Work out the finished part from the listing and answer in its coordinate system (mm). Face numbers are marked on the shaded views. A direction names the side the tool comes from. Give positions to 0.01 mm unless a question says otherwise; leave off trailing zeros. Order: outer loops, then holes, each group sorted by start corner. A loop starts at its lowest first (then second) coordinate and runs counter-clockwise, first axis right, second up.
```python
from build123d import *

# Parameters (mm, degrees)
CYLINDER002_R          = 2
CYLINDER002_DEPTH      = 2
CYLINDER_R             = 1.05
CYLINDER_DEPTH         = 20
CYLINDER_ROLL_ANGLE    = 90
RECTANGLE004_W         = 26
RECTANGLE004_H         = 4.8
EXTRUDE005_DEPTH       = 8
RECTANGLE002_W         = 26
RECTANGLE002_H         = 1
EXTRUDE004_DEPTH       = 20
RECTANGLE005_W         = 26
RECTANGLE005_H         = 4.8
EXTRUDE008_DEPTH       = 8
RECTANGLE001_W         = 26
RECTANGLE001_H         = 1
EXTRUDE002_DEPTH       = 20
RECTANGLE_W            = 27
RECTANGLE_H            = 15
EXTRUDE_DEPTH          = 9
FILLET_R               = 4
FILLET001_R            = 1.8
RECTANGLE008_W         = 26
RECTANGLE008_H         = 4.8
EXTRUDE011_DEPTH       = 8
RECTANGLE007_W         = 26
RECTANGLE007_H         = 1
EXTRUDE010_DEPTH       = 20
RECTANGLE009_W         = 26
RECTANGLE009_H         = 4.8
EXTRUDE012_DEPTH       = 8
RECTANGLE006_W         = 26
RECTANGLE006_H         = 1
EXTRUDE009_DEPTH       = 20
CYLINDER001_R          = 3
CYLINDER001_DEPTH      = 15
CYLINDER001_ROLL_ANGLE = 90
CUT002_ROLL_ANGLE      = 90


with BuildPart() as cylinder002:
    # Cylinder002 → Cylinder002 (new body)
    with BuildSketch(Plane(origin=(-14, -1.5, 18), x_dir=(1, 0, 0), z_dir=(0, 0, 1))):
        Circle(CYLINDER002_R)
    extrude(amount=CYLINDER002_DEPTH)


with BuildPart() as cylinder:
    # Cylinder → Cylinder (new body)
    with BuildSketch(Plane.XY):
        Circle(CYLINDER_R)
    extrude(amount=CYLINDER_DEPTH)


with BuildPart() as cylinder_1:
    # Cylinder roll: moved
    add(cylinder.part.rotate(Axis((0, 0, 0), (1, 0, 0)), CYLINDER_ROLL_ANGLE))


with BuildPart() as cylinder_2:
    # Cylinder placement: moved
    add(cylinder_1.part.moved(Location((-14, 21, 1.5))))


with BuildPart() as extrude005:
    # Rectangle004 → Extrude005 (new body)
    with BuildSketch(Plane(origin=(-23, 13.1, 0), x_dir=(1, 0, 0), z_dir=(0, 0, 1))):
        with Locations((13, 2.4)):
            Rectangle(RECTANGLE004_W, RECTANGLE004_H)
    extrude(amount=-EXTRUDE005_DEPTH)


with BuildPart() as extrude005_1:
    # Extrude005 placement: moved
    add(extrude005.part.moved(Location((0, 0, 11))))


with BuildPart() as extrude004:
    # Rectangle002 → Extrude004 (new body)
    with BuildSketch(Plane(origin=(-23, 10, 0), x_dir=(1, 0, 0), z_dir=(0, 0, 1))):
        with Locations((13, -0.5)):
            Rectangle(RECTANGLE002_W, RECTANGLE002_H)
    extrude(amount=EXTRUDE004_DEPTH)


with BuildPart() as extrude004_1:
    # Extrude004 placement: moved
    add(extrude004.part.moved(Location((0, 0, -4))))


with BuildPart() as extrude008:
    # Rectangle005 → Extrude008 (new body)
    with BuildSketch(Plane(origin=(-23, 11.9, 0), x_dir=(1, 0, 0), z_dir=(0, 0, 1))):
        with Locations((13, -2.4)):
            Rectangle(RECTANGLE005_W, RECTANGLE005_H)
    extrude(amount=EXTRUDE008_DEPTH)


with BuildPart() as extrude008_1:
    # Extrude008 placement: moved
    add(extrude008.part.moved(Location((0, 0, 3))))


with BuildPart() as fusion:
    # Rectangle001 → Extrude002 (new body)
    with BuildSketch(Plane(origin=(-23, 16, 0), x_dir=(1, 0, 0), z_dir=(0, 0, 1))):
        with Locations((13, 0.5)):
            Rectangle(RECTANGLE001_W, RECTANGLE001_H)
    extrude(amount=-EXTRUDE002_DEPTH)


with BuildPart() as fusion_1:
    # Extrude002 placement: moved
    add(fusion.part.moved(Location((0, -1, 10))))

    # Fusion: union Extrude005, Extrude004, Extrude008
    add(extrude005_1.part)
    add(extrude004_1.part)
    add(extrude008_1.part)


with BuildPart() as fillet001:
    # Rectangle → Extrude (new body)
    with BuildSketch(Plane(origin=(-20, 20, 0), x_dir=(1, 0, 0), z_dir=(0, 0, 1))):
        with Locations((13.5, -7.5)):
            Rectangle(RECTANGLE_W, RECTANGLE_H)
    extrude(amount=EXTRUDE_DEPTH)

    # Fillet
    fillet_edges = [fillet001.edges().sort_by_distance(p)[0] for p in [
        (-20, 20, 4.5),
        (7, 20, 4.5),
        (7, 5, 4.5),
        (-20, 5, 4.5),
    ]]
    fillet(fillet_edges, radius=FILLET_R)

    # Cut: cut Fusion
    add(fusion_1.part, mode=Mode.SUBTRACT)

    # Fillet001
    fillet001_edges = [fillet001.edges().sort_by_distance(p)[0] for p in [
        (-8.259972, 17.9, 3),
        (-8.259972, 7.1, 3),
        (-8.5, 11.9, 3),
        (-8.5, 13.1, 3),
    ]]
    fillet(fillet001_edges, radius=FILLET001_R)


with BuildPart() as extrude011:
    # Rectangle008 → Extrude011 (new body)
    with BuildSketch(Plane(origin=(-23, 13.1, 0), x_dir=(1, 0, 0), z_dir=(0, 0, 1))):
        with Locations((13, 2.4)):
            Rectangle(RECTANGLE008_W, RECTANGLE008_H)
    extrude(amount=-EXTRUDE011_DEPTH)


with BuildPart() as extrude011_1:
    # Extrude011 placement: moved
    add(extrude011.part.moved(Location((0, 0, 11))))


with BuildPart() as extrude010:
    # Rectangle007 → Extrude010 (new body)
    with BuildSketch(Plane(origin=(-23, 10, 0), x_dir=(1, 0, 0), z_dir=(0, 0, 1))):
        with Locations((13, -0.5)):
            Rectangle(RECTANGLE007_W, RECTANGLE007_H)
    extrude(amount=EXTRUDE010_DEPTH)


with BuildPart() as extrude010_1:
    # Extrude010 placement: moved
    add(extrude010.part.moved(Location((0, 0, -4))))


with BuildPart() as extrude012:
    # Rectangle009 → Extrude012 (new body)
    with BuildSketch(Plane(origin=(-23, 11.9, 0), x_dir=(1, 0, 0), z_dir=(0, 0, 1))):
        with Locations((13, -2.4)):
            Rectangle(RECTANGLE009_W, RECTANGLE009_H)
    extrude(amount=EXTRUDE012_DEPTH)


with BuildPart() as extrude012_1:
    # Extrude012 placement: moved
    add(extrude012.part.moved(Location((0, 0, 3))))


with BuildPart() as fusion001:
    # Rectangle006 → Extrude009 (new body)
    with BuildSketch(Plane(origin=(-23, 16, 0), x_dir=(1, 0, 0), z_dir=(0, 0, 1))):
        with Locations((13, 0.5)):
            Rectangle(RECTANGLE006_W, RECTANGLE006_H)
    extrude(amount=-EXTRUDE009_DEPTH)


with BuildPart() as fusion001_1:
    # Extrude009 placement: moved
    add(fusion001.part.moved(Location((0, -1, 10))))

    # Fusion001: union Extrude011, Extrude010, Extrude012
    add(extrude011_1.part)
    add(extrude010_1.part)
    add(extrude012_1.part)


with BuildPart() as cut003:
    # Cylinder001 → Cylinder001 (new body)
    with BuildSketch(Plane.XY):
        Circle(CYLINDER001_R)
    extrude(amount=CYLINDER001_DEPTH)


with BuildPart() as cut003_1:
    # Cylinder001 roll: moved
    add(cut003.part.rotate(Axis((0, 0, 0), (1, 0, 0)), CYLINDER001_ROLL_ANGLE))


with BuildPart() as cut003_2:
    # Cylinder001 placement: moved
    add(cut003_1.part.moved(Location((-14, 20, 1.5))))

    # Cut001: cut Fusion001
    add(fusion001_1.part, mode=Mode.SUBTRACT)

    # Fusion002: union Fillet001
    add(fillet001.part)

    # Cut002: cut Cylinder
    add(cylinder_2.part, mode=Mode.SUBTRACT)


with BuildPart() as cut003_3:
    # Cut002 roll: moved
    add(cut003_2.part.rotate(Axis((0, 0, 0), (1, 0, 0)), CUT002_ROLL_ANGLE))


with BuildPart() as cut003_4:
    # Cut002 placement: moved
    add(cut003_3.part)

    # Cut003: cut Cylinder002
    add(cylinder002.part, mode=Mode.SUBTRACT)


solid = cut003_4.part
```
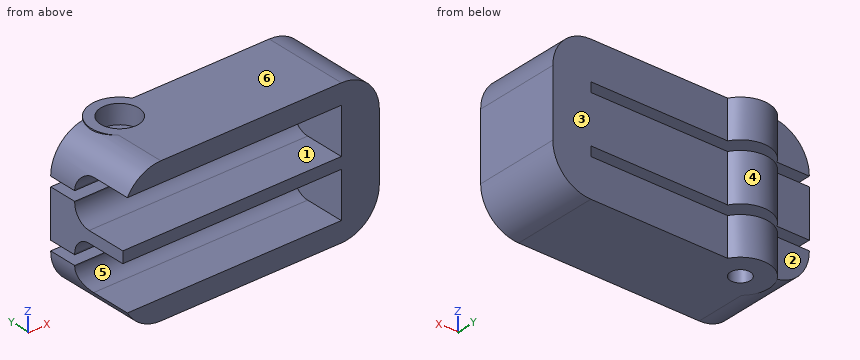
1. Which of the six approach directions +Z, -Z, +X, -X, +Y, -Y give full straight-line access (tool end or side, diameter ignored) to the marked faces 1, 2 and 3?
Findings below:
face 1: -X, -Y
face 2: +Z, -Z, -X, +Y
face 3: +Z, -Z, +X, +Y
2. The part is cut by section C-C (z = 6.5). Write down the section's boundary in (x, y).
Findings below:
outline: (-19.12, -9) - (6.12, -9) - (6.12, 0) - (-11.4, 0) arc R3 ccw to (-16.6, 0) - (-19.12, 0) - close; hole circle Ø2.1 at (-14, -1.5)
3. Straight lines are drawn through the part: probe 1 along Z at (x, y) = (-9.5, -5.25); probe 2 along Z at (x, y) = (-16.25, -1.5); probe 3 along Y at (x, z) = (-14, 7). For each, find the intervals that lie inside material, in ascending order.
Findings below:
probe 1: z = 5 to 7.1, 11.9 to 13.1, 17.9 to 20
probe 2: z = 5 to 9, 10 to 15, 16 to 20
probe 3: y = -9 to -2.55, -0.45 to 1.5
4. The part is cut by section B-B (y = -1.5). State how many separate pieces and enclosed holes the cut face has, then the cut area to 3 significant figures.
Findings below:
separate pieces: 4
enclosed holes: 0
area: 314 mm2
5. The part is cut by section A-A (x = -1). Write down the section's boundary in (y, z), then the cut area to 3 significant figures.
Findings below:
outline: (-9, 5) - (0, 5) - (0, 9) - (-3, 9) - (-3, 8.9) arc R1.8 cw to (-4.8, 7.1) - (-9, 7.1) - close; (-9, 11.9) - (-4.8, 11.9) arc R1.8 cw to (-3, 10.1) - (-3, 10) - (0, 10) - (0, 15) - (-3, 15) - (-3, 14.9) arc R1.8 cw to (-4.8, 13.1) - (-9, 13.1) - close; (-9, 17.9) - (-4.8, 17.9) arc R1.8 cw to (-3, 16.1) - (-3, 16) - (0, 16) - (0, 20) - (-9, 20) - close
area: 74.2 mm2
6. The mould has two halves that part along Z. Classify the marked faces 4, 5 and 6: pulls with the +Z half, pulls with the -Z half, needs draft (parallel to the pull), parting line crosses it, or undercut.
Findings below:
face 4: needs draft
face 5: undercut
face 6: pulls with the +Z half
7. Given P1, Ø2.5, axis at x = -14, y = -1.5, coming from the +Z side; P2, Ø1, axis at x = -19, z = 6.5, coming from the +Y side, each flat-ended and moving along its own axis, determine where each tip first touches the part or whether it passes through.
Findings below:
P1: stops at z = 18
P2: stops at y = 0
